Source: CAD feature listing. Evaluate the final solid. Frame: model axes, mm. Coordinates: 2 decimals unless noted, no trailing zeros. Loops run counter-clockwise (first coordinate to the right, second up) from the corner with the lowest first, then second, coordinate; pieces in that order, holes last.
```python
from build123d import *

# Parameters (mm, degrees)
F0_R     = 25.4
F1_DEPTH = 50.8


with BuildPart() as f1:
    # F0 (on Front) → F1 (new body)
    with BuildSketch(Plane.XZ):
        with BuildLine():
            Line((0, 584.2), (0, 0))
            Line((0, 0), (254, 0))
            Line((254, 0), (254, 584.2))
            ThreePointArc((254, 584.2), (216.802561, 674.002561), (127, 711.2))
            ThreePointArc((127, 711.2), (37.197439, 674.002561), (0, 584.2))
        make_face()
        with Locations((127, 584.2)):
            Circle(F0_R, mode=Mode.SUBTRACT)
    extrude(amount=F1_DEPTH)


solid = f1.part
```
Q1. Section query A-A on y = -26. Return the cut outline in (x, z).
Q2. Section query C-C on x = 210. Return the cut outline in (y, z).
Q3. Draft query along Z for faces 1 (the flat face through (125, -25, 0)), 2 (the cylindrical face through (121.494, -25.044, 559.404)), 3 (the flat face through (125, 0, 361)). Return one class per face: released by +Z, released by -Z, zero draft, split by the parting line, or undercut.
Q4. Section query B-B on x = 108.5. Return the cut outline in (y, z), then the cut area to 3 significant figures.
Q5. First-contact query: pin 1 Ø4 at (y, z) = (-5.5, 482) entering from -X; pin 2 Ø10 at (y, z) = (-14, 626.5) entering from +X. Flat tips, straight axial feed; report the tip coordinate or a pass-through.
Q6. Material intervals for line 1 along Z through (x, y) = (127, -24); line 2 along X through (y, z) = (-28, 584); line 3 along Z through (x, y) = (106.5, -21.5), sorted ascending.
Q7. Section query D-D on z = 656. Return the cut outline in (x, y).
Resolved:
1. outline: (0, 0) - (254, 0) - (254, 584.2) arc R127 ccw to (127, 711.2) arc R127 ccw to (0, 584.2) - close; hole circle Ø50.8 at (127, 584.2)
2. outline: (-50.8, 0) - (0, 0) - (0, 680.32) - (-50.8, 680.32) - close
3. face 1: released by -Z
3. face 2: undercut
3. face 3: zero draft
4. outline: (-50.8, 0) - (0, 0) - (0, 566.8) - (-50.8, 566.8) - close; (-50.8, 601.6) - (0, 601.6) - (0, 709.85) - (-50.8, 709.85) - close
4. area: 34,300 mm2
5. pin 1: stops at x = 0
5. pin 2: stops at x = 248.4
6. line 1: z = 0 to 558.8, 609.6 to 711.2
6. line 2: x = 0 to 101.6, 152.4 to 254
6. line 3: z = 0 to 569.2, 599.2 to 709.53
7. outline: (22.24, -50.8) - (231.76, -50.8) - (231.76, 0) - (22.24, 0) - close
